Here's how the part is built. I have some questions about the finished solid (model axes, mm). A direction names the side the tool comes from. Coordinates: 2 decimals unless noted, no trailing zeros. Loops run counter-clockwise (first coordinate to the right, second up) from the corner with the lowest first, then second, coordinate; pieces in that order, holes last. Notation, with made-up numbers: M 33,-23.5 L 89,-23.5 A26 cw 89,-4.5 Z; hole C 35.5,-35.5 d8. An arc over 180 degrees is marked long. Use one line per item in the form item = value. Start each with the question number.
(1) Imagine slicing it at A-A, the plane x = 12.5. Please give me the cut outline in (y, z).
(2) Imagine slicing it at B-B, the plane y = -2.3. State how many separate pieces and enclosed holes the cut face has, and give its area (3 significant figures).
(3) Please list where these lines run through material, in increasing order: L1, parallel to Z at x = 33, y = -1.8; L2, parallel to Z at x = 44, y = -1.15; L3, parallel to Z at x = 42, y = -0.45.
(4) Will these pins go through, and if not, where does the flat tip stop? P1, Ø4, axis at x = 44.45, z = 0, coming from the +Y side; P2, Ø1.5, axis at x = -7.5, y = -1.5, coming from the +Z side.
(5) Imagine slicing it at D-D, the plane z = 83. Please give me the cut outline in (x, y).
(6) Thinking about a two-plate mould opening in X: for faces 4 (the cylindrical face through (41.28, -1.63, 0.14)), 5 (the cylindrical face through (-15.756, -1.628, 61.558)), 6 (the flat face through (22, -2, -7.938)), which applies, +X half, -X half, draft (parallel to the pull), parting line (faces both ways), or undercut?
(7) On a 3-axis mill with a long thin cutter (end or side, diameter ignored), from which of +Z, -Z, +X, -X, +Y, -Y can I reach the whole of each face in a straight line? I mean faces 1 (the flat face through (31, -2, 7.938)), 2 (the cylindrical face through (15.75, -1.63, 61.51)), 3 (the flat face through (-11.714, -1.628, 30.213)). Say none if no direction works.
(8) Imagine slicing it at C-C, the plane x = 37.5. Please give me the cut outline in (y, z).
```python
from build123d import *

# Parameters (mm, degrees)
F0_R     = 3.175
F1_DEPTH = 3.302


with BuildPart() as f1:
    # F0 (on Front) → F1 (new body)
    with BuildSketch(Plane.XZ):
        with BuildLine():
            ThreePointArc((-9.525, 114.3), (0, 104.775), (9.525, 114.3))
            ThreePointArc((9.525, 114.3), (0, 123.825), (-9.525, 114.3))
        make_face()
        with Locations((0, 114.3)):
            Circle(F0_R, mode=Mode.SUBTRACT)
        with BuildLine():
            Line((15.747457, 65.508289), (9.525, 114.3))
            ThreePointArc((9.525, 114.3), (0, 104.775), (-9.525, 114.3))
            Line((-9.525, 114.3), (-15.747457, 65.508289))
            ThreePointArc((-15.747457, 65.508289), (0, 79.375), (15.747457, 65.508289))
        make_face()
        with Locations((-3.175, 100.0252)):
            Circle(F0_R, mode=Mode.SUBTRACT)
        with BuildLine():
            ThreePointArc((15.875, 63.5), (15.843082, 64.506168), (15.747457, 65.508289))
            ThreePointArc((15.747457, 65.508289), (0, 79.375), (-15.747457, 65.508289))
            ThreePointArc((-15.747457, 65.508289), (-15.843082, 64.506168), (-15.875, 63.5))
            Line((-15.875, 63.5), (-15.386538, 59.592308))
            ThreePointArc((-15.386538, 59.592308), (0.011376, 47.625004), (15.392123, 59.614363))
            Line((15.392123, 59.614363), (15.875, 63.5))
        make_face()
        with Locations((0, 63.5)):
            Circle(F0_R, mode=Mode.SUBTRACT)
        with BuildLine():
            ThreePointArc((15.392123, 59.614363), (15.753818, 61.542237), (15.875, 63.5))
            Line((15.875, 63.5), (15.392123, 59.614363))
        make_face()
        with BuildLine():
            Line((-15.386538, 59.592308), (-15.875, 63.5))
            ThreePointArc((-15.875, 63.5), (-15.752411, 61.530949), (-15.386538, 59.592308))
        make_face()
        with BuildLine():
            Line((10.082594, 16.889395), (15.392123, 59.614363))
            ThreePointArc((15.392123, 59.614363), (0.011376, 47.625004), (-15.386538, 59.592308))
            Line((-15.386538, 59.592308), (-7.9375, 0))
            ThreePointArc((-7.9375, 0), (0, 7.9375), (7.9375, 0))
            ThreePointArc((7.9375, 0), (5.61266, -5.61266), (0, -7.9375))
            Line((0, -7.9375), (44.45, -7.9375))
            ThreePointArc((44.45, -7.9375), (36.5125, 0), (44.45, 7.9375))
            Line((44.45, 7.9375), (17.969436, 7.9375))
            ThreePointArc((17.969436, 7.9375), (12.004147, 10.632131), (10.082594, 16.889395))
        make_face()
        with BuildLine():
            ThreePointArc((7.9375, 0), (0, 7.9375), (-7.9375, 0))
            ThreePointArc((-7.9375, 0), (-5.61266, -5.61266), (0, -7.9375))
            ThreePointArc((0, -7.9375), (5.61266, -5.61266), (7.9375, 0))
        make_face()
        Circle(F0_R, mode=Mode.SUBTRACT)
        with BuildLine():
            ThreePointArc((52.3875, 0), (50.06266, 5.61266), (44.45, 7.9375))
            ThreePointArc((44.45, 7.9375), (36.5125, 0), (44.45, -7.9375))
            ThreePointArc((44.45, -7.9375), (50.06266, -5.61266), (52.3875, 0))
        make_face()
        with Locations((44.45, 0)):
            Circle(F0_R, mode=Mode.SUBTRACT)
    extrude(amount=F1_DEPTH)


solid = f1.part
```
Answer:
q1.outline = M -3.3,-7.94 L 0,-7.94 L 0,10.12 L -3.3,10.12 Z; M -3.3,36.34 L 0,36.34 L 0,90.97 L -3.3,90.97 Z
q2.separate_pieces = 1
q2.enclosed_holes = 5
q2.area = 3,600 mm²
q3.L1 = -7.94 to 7.94
q3.L2 = -7.94 to -3.14, 3.14 to 7.94
q3.L3 = -7.94 to -2.02, 2.02 to 7.94
q4.P1 = through
q4.P2 = 121.02
q5.outline = M -13.52,-3.3 L 13.52,-3.3 L 13.52,0 L -13.52,0 Z
q6.face_4 = undercut
q6.face_5 = -X half
q6.face_6 = draft
q7.face_1 = +Z, +X, +Y, -Y
q7.face_2 = +X, +Y, -Y
q7.face_3 = -Z, -X, +Y, -Y
q8.outline = M -3.3,-7.94 L 0,-7.94 L 0,7.94 L -3.3,7.94 Z
